Design review of the part built by this model. Coordinates are the model's own, in mm. Face numbers are marked on the shaded views. Round coordinates to 2 decimals unless told otherwise and drop trailing zeros. Use one line per item in the form item = value. Start each with the question number.
(1) The part is to be moulded in two halves that separate along Y. For the marked faces 1, 2 and 3, say which applies: released by +Y, released by -Y, zero draft, split by the parting line, or undercut.
(2) Wall thickness on probe 1 along X at (y, z) = (7.5, 6); probe 2 along Z at (x, y) = (-0.25, 15.5); probe 3 along X at (y, z) = (8.5, 2): over which ranges is each line inside the solid? List them lowest first. Write a range as [from, to].
(3) For pin 1 (2 mm diameter, centred on x = -3, z = 2, fed in from -Y); pin 2 (3 mm diameter, centred on x = 4, y = 8.5, fed in from -Z); pin 3 (1 mm diameter, centred on y = 5, z = 4, fed in from +X); pin 4 (2 mm diameter, centred on y = 13, z = 11, fed in from -X), all flat-tipped, find the tip position at first contact; note any pin that passes through.
Autodesk Inventor part; units mm, degrees
ref_plane "YZ Plane" through (0, 0, 0) normal (1, 0, 0) x (0, 1, 0)
ref_plane "XZ Plane" through (0, 0, 0) normal (0, 1, 0) x (-1, 0, 0)
ref_plane "XY Plane" through (0, 0, 0) normal (0, 0, 1) x (1, 0, 0)
sketch "Sketch1" plane through (0, 0, 0) normal (0, 0, 1) x (1, 0, 0)
  line L0 (-0.381, -9.136) -> (-0.381, 8.4693)
  line L1 (-6.477, 0) -> (5.715, 0)
  line L2 (-6.477, 0) -> (-6.477, 27.94)
  line L3 (-6.477, 27.94) -> (5.715, 27.94)
  line L4 (5.715, 27.94) -> (5.715, 0)
  point P0 (0, 0)
  dimension "dw" = 12.192
  dimension "d1" = 6.096
  dimension "d2" = 27.94
extrude "Extrusion1" add sketch "Sketch1" along normal blind 12.192
fillet "Fillet1" radius 6.096 4 edges at (5.715, 13.97, 12.192) (5.715, 13.97, 0) (-6.477, 13.97, 0) (-6.477, 13.97, 12.192)
fillet "Fillet2" radius 1.5875 3 edges at (5.715, 27.94, 6.096) (3.9297, 27.94, 10.4067) (-0.381, 27.94, 12.192)
fillet "Fillet3" radius 1.5875 3 edges at (-0.381, 0, 12.192) (3.9297, 0, 10.4067) (5.715, 0, 6.096)
equation "\"d1\" = 0.5 * dw"
equation "\"d3\" = dw"
equation "\"d5\" = 0.5 * dw"
properties part number "dowel"
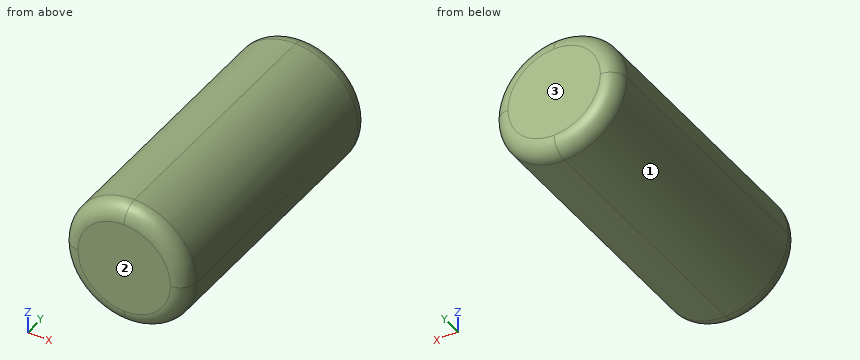
Data:
q1.face_1 = zero draft
q1.face_2 = released by -Y
q1.face_3 = released by +Y
q2.probe_1 = [-6.48, 5.71]
q2.probe_2 = [0, 12.19]
q2.probe_3 = [-4.9, 4.13]
q3.pin_1 = 0
q3.pin_2 = 0.72
q3.pin_3 = 5.5
q3.pin_4 = -5.06
